The figure shows three views and two pictorial views of one solid part (mm, origin at its lowest corner). Answer the questions. A direction names the side the tool comes from. Coordinates: 2 decimals unless noted, no trailing zeros. Write each loop counter-clockwise with the first axis right and the second up, starting at its lowest first coordinate (ties: lowest second). Pieces come first, ordered by that corner, then holes. Notation, with made-up numbers: (22.5, 53) - (69.5, 53) arc R20 ccw to (69.5, 89) - close; hole circle Ø10 at (9, 42.25). An arc over 180 degrees is marked (long way). Use a Markdown table: item, result. Add a question column.
(1) The part is cut by section C-C, the plane y = 9. Give the vertices of the cut face in (x, z).
(2) The part is cut by section B-B, the plane x = 69. Give the vertices of the cut face in (y, z), then the cut area to 3 significant figures.
(3) The part is cut by section A-A, the plane z = 10. Give the vertices of the cut face in (x, y), then the cut area to 3 significant figures.
(4) Given pin 1 Ø3.5 at (y, z) = (4, 25.5) entering from -X, flat-ended and moving along its own axis, determine where the tip first touches the part or whether it passes through.
(5) A tool of negligible diameter and unlimited length cuts with its end or side. For the marked faces 1, 2 and 3, from which of +Z, -Z, +X, -X, +Y, -Y can it reach the whole face along a straight path? Write none if from no direction.
(6) The part is cut by section D-D, the plane x = 79. Give the vertices of the cut face in (y, z), then the cut area to 3 significant figures.
(7) Find the intervals of material crossed by line 1 (X direction, y = 6, z = 10); line 2 (Z direction, x = 68.5, y = 8.5); line 3 (X direction, y = 2.5, z = 35.5), in increasing order. Write a range as from..to.
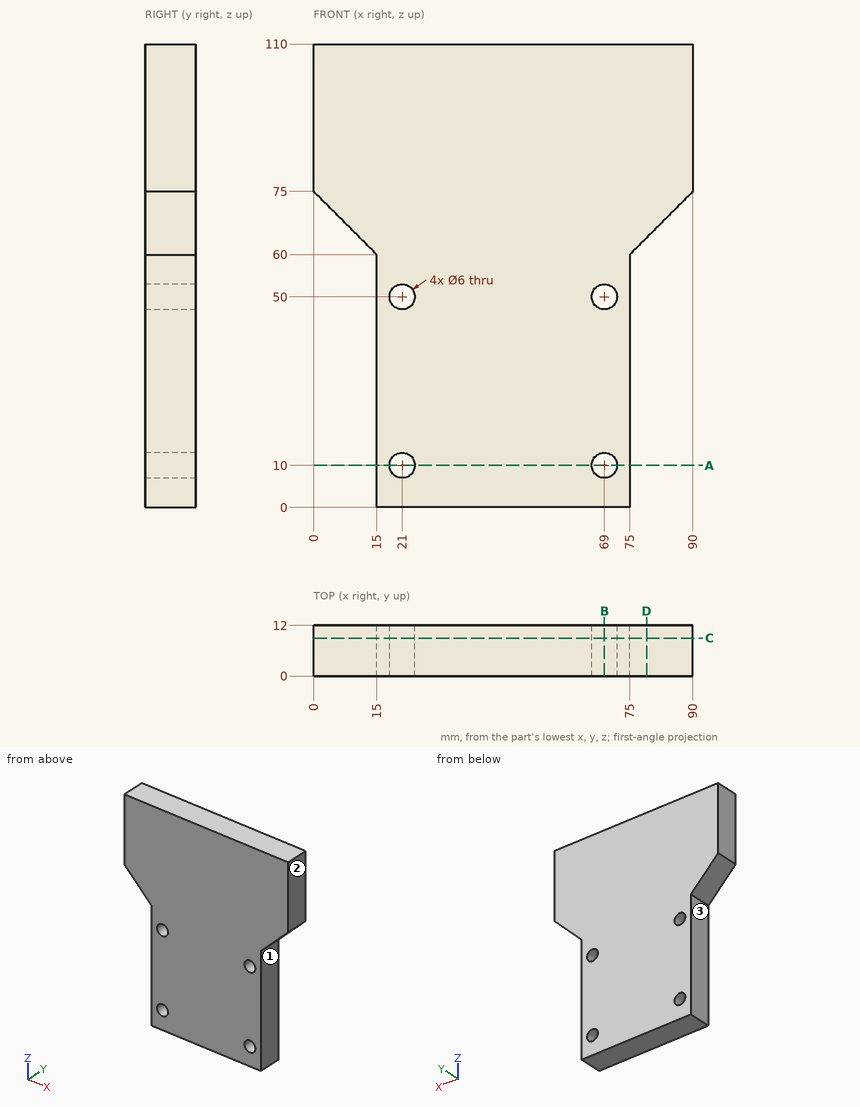
Model answer:
| question | item | result |
|---|---|---|
| 1 | outline | (0, 75) - (15, 60) - (15, 0) - (75, 0) - (75, 60) - (90, 75) - (90, 110) - (0, 110) - close; hole circle Ø6 at (21, 10); hole circle Ø6 at (21, 50); hole circle Ø6 at (69, 10); hole circle Ø6 at (69, 50) |
| 2 | outline | (0, 0) - (12, 0) - (12, 7) - (0, 7) - close; (0, 13) - (12, 13) - (12, 47) - (0, 47) - close; (0, 53) - (12, 53) - (12, 110) - (0, 110) - close |
| 2 | area | 1,180 mm^2 |
| 3 | outline | (15, 0) - (18, 0) - (18, 12) - (15, 12) - close; (24, 0) - (66, 0) - (66, 12) - (24, 12) - close; (72, 0) - (75, 0) - (75, 12) - (72, 12) - close |
| 3 | area | 576 mm^2 |
| 4 | pin 1 | x = 15 |
| 5 | face 1 | -Z, +X, +Y, -Y |
| 5 | face 2 | +Z, -Z, +X, +Y, -Y |
| 5 | face 3 | -Z, -X, +Y, -Y |
| 6 | outline | (0, 64) - (12, 64) - (12, 110) - (0, 110) - close |
| 6 | area | 552 mm^2 |
| 7 | line 1 | 15..18, 24..66, 72..75 |
| 7 | line 2 | 0..7.04, 12.96..47.04, 52.96..110 |
| 7 | line 3 | 15..75 |
